Geometry: final body of the model. Coordinates: model frame, mm. A direction names the side the tool comes from. Coordinates: 2 decimals unless noted, no trailing zeros. Write each loop counter-clockwise with the first axis right and the second up, starting at its lowest first coordinate (ties: lowest second). Pieces come first, ordered by that corner, then holes. Notation, with made-up numbers: (-5.5, 33) - (52.5, 33) arc R37 ccw to (52.5, 72) - close; hole circle Ø3 at (80.5, 20). An arc over 180 degrees is marked (long way). Put each result on its own line as item: value.
```python
from build123d import *

# Parameters (mm, degrees)
F0_R     = 18
F1_DEPTH = 0.5
F2_R     = 4.05
F3_DEPTH = 0.5
F5_DEPTH = 0.5


with BuildPart() as f1:
    # F0 (on Top) → F1 (new body)
    with BuildSketch(Plane.XY):
        Circle(F0_R)
    extrude(amount=F1_DEPTH)

    # F2 (on face) → F3 (cut, through all)
    with BuildSketch(Plane.XY.offset(0.5)):
        Circle(F2_R)
    extrude(amount=-F3_DEPTH, mode=Mode.SUBTRACT)

    # F4 (on face) → F5 (cut, through all)
    with BuildSketch(Plane.XY.offset(0.5)):
        with BuildLine():
            Line((-1, -13.462912), (-1, -5.408327))
            ThreePointArc((-1, -5.408327), (-3.889087, -3.889087), (-5.408327, -1))
            Line((-5.408327, -1), (-13.462912, -1))
            ThreePointArc((-13.462912, -1), (-9.545942, -9.545942), (-1, -13.462912))
        make_face()
        with BuildLine():
            Line((13.462912, -1), (5.408327, -1))
            ThreePointArc((5.408327, -1), (3.889087, -3.889087), (1, -5.408327))
            Line((1, -5.408327), (1, -13.462912))
            ThreePointArc((1, -13.462912), (9.545942, -9.545942), (13.462912, -1))
        make_face()
        with BuildLine():
            ThreePointArc((1, 5.408327), (3.889087, 3.889087), (5.408327, 1))
            Line((5.408327, 1), (13.462912, 1))
            ThreePointArc((13.462912, 1), (9.545942, 9.545942), (1, 13.462912))
            Line((1, 13.462912), (1, 5.408327))
        make_face()
        with BuildLine():
            ThreePointArc((-5.408327, 1), (-3.889087, 3.889087), (-1, 5.408327))
            Line((-1, 5.408327), (-1, 13.462912))
            ThreePointArc((-1, 13.462912), (-9.545942, 9.545942), (-13.462912, 1))
            Line((-13.462912, 1), (-5.408327, 1))
        make_face()
    extrude(amount=-F5_DEPTH, mode=Mode.SUBTRACT)


solid = f1.part
```
1. Set-up query: faces 1 (the flat face through (3.7, -3.7, 0.5)), 2 (the cylindrical face through (-3.86, -3.92, 0.25)). Return all of +Z, -Z, +X, -X, +Y, -Y with unobstructed straight access to the full face (end or side cutting, diameter ignored); none if empty.
Answer below:
face 1: +Z, +X, -X, +Y, -Y
face 2: +Z, -Z
2. Section query B-B (y = 0). Return loops of the section in (x, z), then the cut area to 4 significant figures.
Answer below:
outline: (-18, 0) - (-4.05, 0) - (-4.05, 0.5) - (-18, 0.5) - close; (4.05, 0) - (18, 0) - (18, 0.5) - (4.05, 0.5) - close
area: 13.95 mm²
3. Ray query, probe 1 along Y at (x, z) = (0, 0.25); probe 2 along Y at (x, z) = (-8, 0.15); probe 3 along X at (y, z) = (-9, 0.2). Return the intervals inside material, ascending. Write a range as from..to.
Answer below:
probe 1: y = -18..-4.05, 4.05..18
probe 2: y = -16.12..-10.87, -1..1, 10.87..16.12
probe 3: x = -15.59..-10.06, -1..1, 10.06..15.59
4. Mould query, pull axis X, two halves, no side actions, for faces 3 (the cylindrical face through (-9.64, -9.45, 0.25)), 4 (the flat face through (3.7, -3.7, 0)), 5 (the cylindrical face through (-2.343, 17.847, 0.246)). Classes: +X half, -X half, draft (parallel to the pull), parting line (faces both ways), or undercut.
Answer below:
face 3: undercut
face 4: draft
face 5: parting line
5. Section query A-A (z = 0.3). Return loops of the section in (x, y), then the cut area to 3 significant figures.
Answer below:
outline: circle Ø36 at (0, 0); hole (-13.46, -1) arc R13.5 ccw to (-1, -13.46) - (-1, -5.41) arc R5.5 cw to (-5.41, -1) - close; hole (-13.46, 1) - (-5.41, 1) arc R5.5 cw to (-1, 5.41) - (-1, 13.46) arc R13.5 ccw to start; hole circle Ø8.1 at (0, 0); hole (1, -13.46) arc R13.5 ccw to (13.46, -1) - (5.41, -1) arc R5.5 cw to (1, -5.41) - close; hole (1, 5.41) arc R5.5 cw to (5.41, 1) - (13.46, 1) arc R13.5 ccw to (1, 13.46) - close
area: 553 mm²
6. Section query D-D (y = 9). Return loops of the section in (x, z), then the cut area to 3 significant figures.
Answer below:
outline: (-15.59, 0) - (-10.06, 0) - (-10.06, 0.5) - (-15.59, 0.5) - close; (-1, 0) - (1, 0) - (1, 0.5) - (-1, 0.5) - close; (10.06, 0) - (15.59, 0) - (15.59, 0.5) - (10.06, 0.5) - close
area: 6.53 mm²
